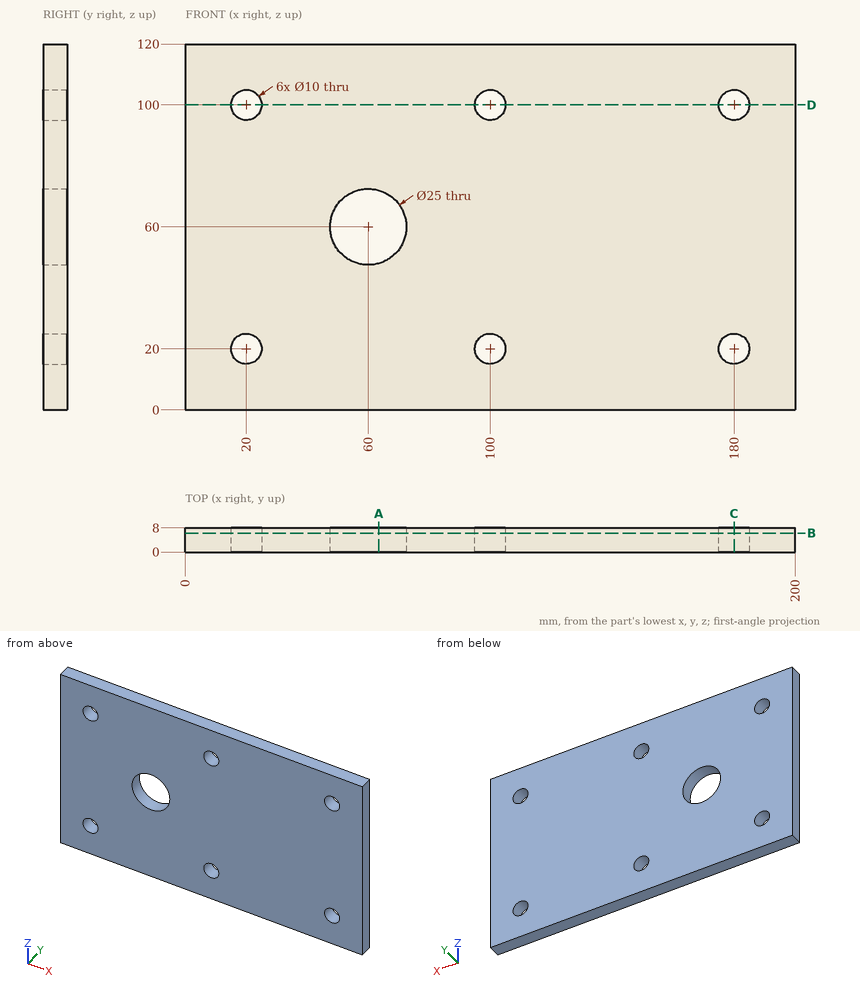
Study the drawing (mm; zero at the part's minimum x, y, z) and answer. Give positions to 0.01 mm unless a question says otherwise; leave off trailing zeros. Write each loop counter-clockwise with the first axis right and the second up, starting at its lowest first coordinate (ties: lowest second). Pieces come first, ordered by that corner, then holes.
(1) Straight lines are drawn through the part: line 1 (X direction, y = 3.5, z = 100); line 2 (Z direction, x = 20, y = 4); line 3 (X direction, y = 3.5, z = 104.5). For each, find the intervals that lie inside material, in ascending order.
Final values:
line 1: x = 0 to 15, 25 to 95, 105 to 175, 185 to 200
line 2: z = 0 to 15, 25 to 95, 105 to 120
line 3: x = 0 to 17.82, 22.18 to 97.82, 102.18 to 177.82, 182.18 to 200
(2) A flat-ended cylindrical pin translates along its axis: pin 1 Ø6 at (x, z) = (20, 100) entering from +Y. Find the tip coordinate at first contact, or state that the pin passes through.
Final values:
pin 1: passes through
(3) The part is cut by section C-C on x = 180. Write down the section's boundary in (y, z).
Final values:
outline: (0, 0) - (8, 0) - (8, 15) - (0, 15) - close; (0, 25) - (8, 25) - (8, 95) - (0, 95) - close; (0, 105) - (8, 105) - (8, 120) - (0, 120) - close
(4) The part is cut by section D-D on z = 100. Write down the section's boundary in (x, y).
Final values:
outline: (0, 0) - (15, 0) - (15, 8) - (0, 8) - close; (25, 0) - (95, 0) - (95, 8) - (25, 8) - close; (105, 0) - (175, 0) - (175, 8) - (105, 8) - close; (185, 0) - (200, 0) - (200, 8) - (185, 8) - close
(5) The part is cut by section B-B on y = 6.25. Write down the section's boundary in (x, z).
Final values:
outline: (0, 0) - (200, 0) - (200, 120) - (0, 120) - close; hole circle Ø10 at (20, 20); hole circle Ø10 at (20, 100); hole circle Ø25 at (60, 60); hole circle Ø10 at (100, 20); hole circle Ø10 at (100, 100); hole circle Ø10 at (180, 20); hole circle Ø10 at (180, 100)
(6) The part is cut by section A-A on x = 63.5. Write down the section's boundary in (y, z), plus the area to 3 significant figures.
Final values:
outline: (0, 0) - (8, 0) - (8, 48) - (0, 48) - close; (0, 72) - (8, 72) - (8, 120) - (0, 120) - close
area: 768 mm2
